from build123d import *

# Parameters (mm, degrees)
BOSS_EXTRUDE1_DEPTH = 5.08
SKETCH2_W           = 25.4
SKETCH2_H           = 0.8334375
CUT_EXTRUDE1_DEPTH  = 13.97
SKETCH3_R           = 1.4224
CUT_EXTRUDE2_DEPTH  = 12.7
CUT_EXTRUDE3_DEPTH  = 12.7
FILLET3_R           = 5.08


with BuildPart() as part:
    # Sketch1 → Boss-Extrude1 (new body)
    with BuildSketch(Plane(origin=(0, 0, 0), x_dir=(1, 0, 0), z_dir=(0, 1, 0))):
        Polygon((-33.096969697, 5.387878788), (-20.396969697, 5.387878788), (-4.521969697, 5.387878788), (-4.521969697, -0.962121212), (-20.396969697, -0.962121212), (-20.396969697, -20.012121212), (-33.096969697, -20.012121212), align=None)
    extrude(amount=BOSS_EXTRUDE1_DEPTH)

    # Sketch2 → Cut-Extrude1 (cut)
    with BuildSketch(Plane.ZY.offset(33.096969697)):
        with Locations((7.312121212, 2.54)):
            Rectangle(SKETCH2_W, SKETCH2_H)
    extrude(amount=-CUT_EXTRUDE1_DEPTH, mode=Mode.SUBTRACT)

    # Sketch3 → Cut-Extrude2 (cut)
    with BuildSketch(Plane(origin=(0, 5.08, 0), x_dir=(1, 0, 0), z_dir=(0, 1, 0))):
        with Locations(Location((-26.746969697, -16.837121212, 0), (0, 0, 90))):
            Circle(SKETCH3_R)
        with Locations(Location((-26.746969697, -10.487121212, 0), (0, 0, 90))):
            Circle(SKETCH3_R)
        with Locations(Location((-26.746969697, -4.137121212, 0), (0, 0, 90))):
            Circle(SKETCH3_R)
        with Locations(Location((-26.746969697, 2.212878788, 0), (0, 0, 90))):
            Circle(SKETCH3_R)
    extrude(amount=-CUT_EXTRUDE2_DEPTH, mode=Mode.SUBTRACT)

    # Sketch5 → Cut-Extrude3 (cut)
    with BuildSketch(Plane.XY.offset(0.962121212)):
        with BuildLine():
            Line((-6.579369697, 1.290485214), (-6.579369697, 3.789514786))
            ThreePointArc((-6.579369697, 3.789514786), (-9.373369697, 2.54), (-6.579369697, 1.290485214))
        make_face()
    extrude(amount=-CUT_EXTRUDE3_DEPTH, mode=Mode.SUBTRACT)

    # Fillet3
    # the kernel refuses this fillet: 5.08 mm, written as the material it adds along each edge
    with BuildSketch(Plane(origin=(-20.396969697, -9.74328125, 0.962121212), x_dir=(1, 0, 0), z_dir=(0, 1, 0))) as fillet3_piece_1_section:
        with BuildLine():
            CenterArc((FILLET3_R, -FILLET3_R), FILLET3_R, 90, 90)
            Line((0, -FILLET3_R), (0, 0))
            Line((0, 0), (FILLET3_R, 0))
        make_face()
    fillet3_piece_1 = extrude(amount=14.82328125, mode=Mode.PRIVATE)
    fillet3_piece_1 = split(fillet3_piece_1, bisect_by=Plane(origin=(-18.050290176, 0, 1.370319311), z_dir=(0, 1, 0)), keep=Keep.TOP, mode=Mode.PRIVATE)
    fillet3_piece_1 = split(fillet3_piece_1, bisect_by=Plane(origin=(-18.050290176, 2.12328125, 1.370319311), z_dir=(0, -1, 0)), keep=Keep.TOP, mode=Mode.PRIVATE)
    fillet3_piece_1 = split(fillet3_piece_1, bisect_by=Plane(origin=(-19.126969697, 1.061640625, 1.370319311), z_dir=(1, 0, 0)), keep=Keep.TOP, mode=Mode.PRIVATE)
    add(fillet3_piece_1)
    with BuildSketch(Plane(origin=(-20.396969697, -9.74328125, 0.962121212), x_dir=(1, 0, 0), z_dir=(0, 1, 0))) as fillet3_piece_2_section:
        with BuildLine():
            CenterArc((FILLET3_R, -FILLET3_R), FILLET3_R, 90, 90)
            Line((0, -FILLET3_R), (0, 0))
            Line((0, 0), (FILLET3_R, 0))
        make_face()
    fillet3_piece_2 = extrude(amount=14.82328125, mode=Mode.PRIVATE)
    fillet3_piece_2 = split(fillet3_piece_2, bisect_by=Plane(origin=(-19.932991251, 0, 2.537596858), z_dir=(0, 1, 0)), keep=Keep.TOP, mode=Mode.PRIVATE)
    fillet3_piece_2 = split(fillet3_piece_2, bisect_by=Plane(origin=(-19.932991251, 2.12328125, 2.537596858), z_dir=(0, -1, 0)), keep=Keep.TOP, mode=Mode.PRIVATE)
    fillet3_piece_2 = split(fillet3_piece_2, bisect_by=Plane(origin=(-19.126969697, 1.061640625, 2.537596858), z_dir=(-1, 0, 0)), keep=Keep.TOP, mode=Mode.PRIVATE)
    add(fillet3_piece_2)
    with BuildSketch(Plane(origin=(-20.396969697, -9.74328125, 0.962121212), x_dir=(1, 0, 0), z_dir=(0, 1, 0))) as fillet3_piece_3_section:
        with BuildLine():
            CenterArc((FILLET3_R, -FILLET3_R), FILLET3_R, 90, 90)
            Line((0, -FILLET3_R), (0, 0))
            Line((0, 0), (FILLET3_R, 0))
        make_face()
    fillet3_piece_3 = extrude(amount=14.82328125, mode=Mode.PRIVATE)
    fillet3_piece_3 = split(fillet3_piece_3, bisect_by=Plane(origin=(-18.050290176, 2.12328125, 1.370319311), z_dir=(0, 1, 0)), keep=Keep.TOP, mode=Mode.PRIVATE)
    fillet3_piece_3 = split(fillet3_piece_3, bisect_by=Plane(origin=(-19.126969697, 2.54, 1.370319311), z_dir=(1, 0, 0)), keep=Keep.TOP, mode=Mode.PRIVATE)
    fillet3_piece_3 = split(fillet3_piece_3, bisect_by=Plane(origin=(-18.050290176, 2.95671875, 1.370319311), z_dir=(0, -1, 0)), keep=Keep.TOP, mode=Mode.PRIVATE)
    add(fillet3_piece_3)
    with BuildSketch(Plane(origin=(-20.396969697, 2.95671875, 0.962121212), x_dir=(1, 0, 0), z_dir=(0, 1, 0))) as fillet3_piece_4_section:
        with BuildLine():
            CenterArc((FILLET3_R, -FILLET3_R), FILLET3_R, 90, 90)
            Line((0, -FILLET3_R), (0, 0))
            Line((0, 0), (FILLET3_R, 0))
        make_face()
    fillet3_piece_4 = extrude(amount=2.12328125, mode=Mode.PRIVATE)
    fillet3_piece_4 = split(fillet3_piece_4, bisect_by=Plane(origin=(-19.126969697, 4.018359375, 1.370319311), z_dir=(1, 0, 0)), keep=Keep.TOP, mode=Mode.PRIVATE)
    add(fillet3_piece_4)
    with BuildSketch(Plane(origin=(-20.396969697, 2.95671875, 0.962121212), x_dir=(1, 0, 0), z_dir=(0, 1, 0))) as fillet3_piece_5_section:
        with BuildLine():
            CenterArc((FILLET3_R, -FILLET3_R), FILLET3_R, 90, 90)
            Line((0, -FILLET3_R), (0, 0))
            Line((0, 0), (FILLET3_R, 0))
        make_face()
    fillet3_piece_5 = extrude(amount=2.12328125, mode=Mode.PRIVATE)
    fillet3_piece_5 = split(fillet3_piece_5, bisect_by=Plane(origin=(-19.126969697, 4.018359375, 2.537596858), z_dir=(-1, 0, 0)), keep=Keep.TOP, mode=Mode.PRIVATE)
    add(fillet3_piece_5)
    with BuildSketch(Plane(origin=(-20.396969697, 0, 0.962121212), x_dir=(1, 0, 0), z_dir=(0, 1, 0))) as fillet3_piece_6_section:
        with BuildLine():
            CenterArc((FILLET3_R, -FILLET3_R), FILLET3_R, 90, 90)
            Line((0, -FILLET3_R), (0, 0))
            Line((0, 0), (FILLET3_R, 0))
        make_face()
    fillet3_piece_6 = extrude(amount=2.12328125, mode=Mode.PRIVATE)
    fillet3_piece_6 = split(fillet3_piece_6, bisect_by=Plane(origin=(-19.126969697, 1.061640625, 1.370319311), z_dir=(1, 0, 0)), keep=Keep.TOP, mode=Mode.PRIVATE)
    add(fillet3_piece_6)
    with BuildSketch(Plane(origin=(-20.396969697, 0, 0.962121212), x_dir=(1, 0, 0), z_dir=(0, 1, 0))) as fillet3_piece_7_section:
        with BuildLine():
            CenterArc((FILLET3_R, -FILLET3_R), FILLET3_R, 90, 90)
            Line((0, -FILLET3_R), (0, 0))
            Line((0, 0), (FILLET3_R, 0))
        make_face()
    fillet3_piece_7 = extrude(amount=2.12328125, mode=Mode.PRIVATE)
    fillet3_piece_7 = split(fillet3_piece_7, bisect_by=Plane(origin=(-19.126969697, 1.061640625, 2.537596858), z_dir=(-1, 0, 0)), keep=Keep.TOP, mode=Mode.PRIVATE)
    add(fillet3_piece_7)
    with BuildSketch(Plane(origin=(-20.396969697, 0, 0.962121212), x_dir=(1, 0, 0), z_dir=(0, 1, 0))) as fillet3_piece_8_section:
        with BuildLine():
            CenterArc((FILLET3_R, -FILLET3_R), FILLET3_R, 90, 90)
            Line((0, -FILLET3_R), (0, 0))
            Line((0, 0), (FILLET3_R, 0))
        make_face()
    fillet3_piece_8 = extrude(amount=14.82328125, mode=Mode.PRIVATE)
    fillet3_piece_8 = split(fillet3_piece_8, bisect_by=Plane(origin=(-18.050290176, 2.12328125, 1.370319311), z_dir=(0, 1, 0)), keep=Keep.TOP, mode=Mode.PRIVATE)
    fillet3_piece_8 = split(fillet3_piece_8, bisect_by=Plane(origin=(-19.126969697, 2.54, 1.370319311), z_dir=(1, 0, 0)), keep=Keep.TOP, mode=Mode.PRIVATE)
    fillet3_piece_8 = split(fillet3_piece_8, bisect_by=Plane(origin=(-18.050290176, 2.95671875, 1.370319311), z_dir=(0, -1, 0)), keep=Keep.TOP, mode=Mode.PRIVATE)
    add(fillet3_piece_8)
    with BuildSketch(Plane(origin=(-20.396969697, 0, 0.962121212), x_dir=(1, 0, 0), z_dir=(0, 1, 0))) as fillet3_piece_9_section:
        with BuildLine():
            CenterArc((FILLET3_R, -FILLET3_R), FILLET3_R, 90, 90)
            Line((0, -FILLET3_R), (0, 0))
            Line((0, 0), (FILLET3_R, 0))
        make_face()
    fillet3_piece_9 = extrude(amount=14.82328125, mode=Mode.PRIVATE)
    fillet3_piece_9 = split(fillet3_piece_9, bisect_by=Plane(origin=(-18.050290176, 5.08, 1.370319311), z_dir=(0, -1, 0)), keep=Keep.TOP, mode=Mode.PRIVATE)
    fillet3_piece_9 = split(fillet3_piece_9, bisect_by=Plane(origin=(-19.126969697, 4.018359375, 1.370319311), z_dir=(1, 0, 0)), keep=Keep.TOP, mode=Mode.PRIVATE)
    fillet3_piece_9 = split(fillet3_piece_9, bisect_by=Plane(origin=(-18.050290176, 2.95671875, 1.370319311), z_dir=(0, 1, 0)), keep=Keep.TOP, mode=Mode.PRIVATE)
    add(fillet3_piece_9)
    with BuildSketch(Plane(origin=(-20.396969697, 0, 0.962121212), x_dir=(1, 0, 0), z_dir=(0, 1, 0))) as fillet3_piece_10_section:
        with BuildLine():
            CenterArc((FILLET3_R, -FILLET3_R), FILLET3_R, 90, 90)
            Line((0, -FILLET3_R), (0, 0))
            Line((0, 0), (FILLET3_R, 0))
        make_face()
    fillet3_piece_10 = extrude(amount=14.82328125, mode=Mode.PRIVATE)
    fillet3_piece_10 = split(fillet3_piece_10, bisect_by=Plane(origin=(-19.932991251, 5.08, 2.537596858), z_dir=(0, -1, 0)), keep=Keep.TOP, mode=Mode.PRIVATE)
    fillet3_piece_10 = split(fillet3_piece_10, bisect_by=Plane(origin=(-19.126969697, 4.018359375, 2.537596858), z_dir=(-1, 0, 0)), keep=Keep.TOP, mode=Mode.PRIVATE)
    fillet3_piece_10 = split(fillet3_piece_10, bisect_by=Plane(origin=(-19.932991251, 2.95671875, 2.537596858), z_dir=(0, 1, 0)), keep=Keep.TOP, mode=Mode.PRIVATE)
    add(fillet3_piece_10)


solid = part.part
Work out the finished part from the listing and answer in its coordinate system (mm). A direction names the side the tool comes from. Coordinates: 2 decimals unless noted, no trailing zeros. Write each loop counter-clockwise with the first axis right and the second up, starting at its lowest first coordinate (ties: lowest second). Pieces come first, ordered by that corner, then holes.
1. The part is cut by section A-A, the plane x = -22.25. Write down the section's boundary in (y, z), and give its area (3 significant figures).
Results list:
outline: (0, -5.39) - (2.12, -5.39) - (2.12, 20.01) - (0, 20.01) - close; (2.96, -5.39) - (5.08, -5.39) - (5.08, 20.01) - (2.96, 20.01) - close
area: 108 mm2
2. For a pull along X with two mould halves and no side action, classify faces 4 (the flat face through (-20.397, 4, 13)), 5 (the flat face through (-33.097, 1, 7)), 6 (the cylindrical face through (-25.36, 4.03, -1.9)) as +X half, -X half, draft (parallel to the pull), parting line (faces both ways), or undercut.
Results list:
face 4: +X half
face 5: -X half
face 6: undercut
3. For faces 1 (the flat face through (-26, 2.123, 7)), 2 (the flat face through (-10, 3, 0.962)), 3 (the flat face through (-27, 1, 20.012)), determine the directions among +Z, -Z, +X, -X, +Y, -Y from which every point of the face is accessible in a straight line to the end or side of a thin tool.
Results list:
face 1: +Z, -Z, -X
face 2: +Z, +X, +Y, -Y
face 3: +Z, +X, -X, +Y, -Y
4. The part is cut by section D-D, the plane z = -2. Write down the section's boundary in (x, y).
Results list:
outline: (-33.1, 0) - (-28.15, 0) - (-28.15, 2.12) - (-33.1, 2.12) - close; (-33.1, 2.96) - (-28.15, 2.96) - (-28.15, 5.08) - (-33.1, 5.08) - close; (-25.34, 0) - (-4.52, 0) - (-4.52, 5.08) - (-25.34, 5.08) - (-25.34, 2.96) - (-19.13, 2.96) - (-19.13, 2.12) - (-25.34, 2.12) - close; hole (-6.58, 1.29) - (-6.58, 3.79) arc R1.68 ccw (long way) to start
5. Flat-ended cylindrical pins translate along their axes: pin 1 (1.7 mm diameter, centred on y = 4.5, z = 16, fed in from +X); pin 2 (1.5 mm diameter, centred on x = -12.5, y = 1.5, fed in from +Z). Find the tip coordinate at first contact, or state that the pin passes through.
Results list:
pin 1: stops at x = -20.4
pin 2: stops at z = 0.96
6. Consider line 1 along Y through (x, z) = (-32, 3.5); line 2 along Z through (x, y) = (-27.25, 0.55); line 3 along Z through (x, y) = (-9.75, 1.9). Determine where each line is inside the solid, lowest interval first.
Results list:
line 1: y = 0 to 2.12, 2.96 to 5.08
line 2: z = -5.39 to -3.54, -0.88 to 2.81, 5.47 to 9.16, 11.82 to 15.51, 18.17 to 20.01
line 3: z = -5.39 to 0.96
7. The part is cut by section B-B, the plane y = 2.54. Write down the section's boundary in (x, z), and give its area (3 significant figures).
Results list:
outline: (-19.13, -5.39) - (-9.37, -5.39) - (-9.37, 0.96) - (-15.32, 0.96) arc R5.08 cw to (-19.13, 2.68) - close; (-6.58, -5.39) - (-4.52, -5.39) - (-4.52, 0.96) - (-6.58, 0.96) - close
area: 77.0 mm2
8. The part is cut by section C-C, the plane z = 12.25. Write down the section's boundary in (x, y), and give its area (3 significant figures).
Results list:
outline: (-33.1, 0) - (-20.4, 0) - (-20.4, 2.12) - (-33.1, 2.12) - close; (-33.1, 2.96) - (-20.4, 2.96) - (-20.4, 5.08) - (-33.1, 5.08) - close
area: 53.9 mm2
